Autodesk Inventor part; units mm, degrees
ref_plane "YZ Plane" through (0, 0, 0) normal (1, 0, 0) x (0, 1, 0)
ref_plane "XZ Plane" through (0, 0, 0) normal (0, 1, 0) x (-1, 0, 0)
ref_plane "XY Plane" through (0, 0, 0) normal (0, 0, 1) x (1, 0, 0)
sketch "Esquisse1" plane through (0, 0, 0) normal (0, 1, 0) x (-1, 0, 0)
  circle A0 centre (0, 0) radius 38
  dimension "d0" = 76
extrude "Extrusion1" add sketch "Esquisse1" along normal blind 25
fillet "Congé1" radius 2 1 edges at (38, 25, 0)
fillet "Congé2" radius 2 1 edges at (38, 0, 0)
properties part number "palet"
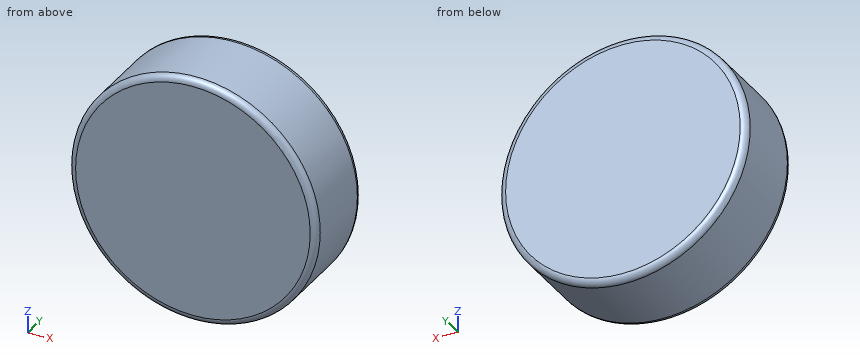
The model under review builds one solid part; all positions refer to its coordinate system, in mm. Round coordinates to 2 decimals unless told otherwise and drop trailing zeros. Order: outer loops, then holes, each group sorted by start corner. A loop starts at its lowest first (then second) coordinate and runs counter-clockwise, first axis right, second up. Notation, with made-up numbers: (33, 46) -> (72, 46) arc R14 cw to (72, 53) -> close; hole circle Ø1 at (11.5, 47). An arc over 180 degrees is marked (long way). Return JSON: item names as keys, results as strings.
1. Insertion check: P1, Ø12, axis at x = -7.5, y = 9.5, coming from the +Z side; P2, Ø5, axis at y = 9.5, z = 23, coming from the -X side; P3, Ø4, axis at y = 19, z = -23.5, coming from the +X side. Each pin has a flat end and moves straight along its axis. Give the tip position at first contact, or say it passes through.
Answer block:
{"P1": "stops at z = 37.97", "P2": "stops at x = -32", "P3": "stops at x = 31.33"}
2. Take a section at A-A (y = 22). Write out the cut boundary in (x, z), then the cut area to 3 significant figures.
Answer block:
{"outline": "circle Ø76 at (0, 0)", "area": "4,540 mm²"}
3. For L1, parallel to X at y = 4.25, z = 17; L2, parallel to X at y = 5.5, z = -1.5; L3, parallel to Z at x = -12.5, y = 14, list the stretches that pass through material, from the lowest coordinate up. Write a range as [from, to].
Answer block:
{"L1": "x = [-33.99, 33.99]", "L2": "x = [-37.97, 37.97]", "L3": "z = [-35.89, 35.89]"}
